```python
from build123d import *

# Parameters (mm, degrees)
BOSS_EXTRUDE1_DEPTH = 115
SKETCH2_R           = 2
CUT_EXTRUDE1_DEPTH  = 243.744721879
SKETCH3_R           = 15.5
CUT_EXTRUDE2_DEPTH  = 60


with BuildPart() as part:
    # Sketch1 → Boss-Extrude1 (new body)
    with BuildSketch(Plane.XY):
        Polygon((0, 0), (0, 40), (-5, 40), (-5, -210), (35, -210), (35, 0), align=None)
    extrude(amount=BOSS_EXTRUDE1_DEPTH)

    # Sketch2 → Cut-Extrude1 (cut, through all)
    with BuildSketch(Plane.ZY.offset(5)):
        with Locations(Location((106, 34, 0), (0, 0, 270))):
            Circle(SKETCH2_R)
        with Locations(Location((66, 34, 0), (0, 0, 270))):
            Circle(SKETCH2_R)
        with Locations((66, 6)):
            Circle(SKETCH2_R)
        with Locations((106, 6)):
            Circle(SKETCH2_R)
    extrude(amount=-CUT_EXTRUDE1_DEPTH, mode=Mode.SUBTRACT)

    # Sketch3 → Cut-Extrude2 (cut)
    with BuildSketch(Plane(origin=(0, 0, 0), x_dir=(-1, 0, 0), z_dir=(0, 0, -1))):
        with Locations((-12, 20)):
            Circle(SKETCH3_R)
    extrude(amount=-CUT_EXTRUDE2_DEPTH, mode=Mode.SUBTRACT)


solid = part.part
```
Model file for the job. Use its own axes, mm. A direction names the side the tool comes from. Give positions to 0.01 mm unless a question says otherwise; leave off trailing zeros. Write each loop counter-clockwise with the first axis right and the second up, starting at its lowest first coordinate (ties: lowest second). Pieces come first, ordered by that corner, then holes. Notation, with made-up numbers: (25.5, -2) - (53.5, -2) arc R13 cw to (53.5, 18) - close; hole circle Ø1 at (-14, 68.5). An arc over 180 degrees is marked (long way). One line per question, with ' | ' between items. Start each with the question number.
(1) Pin check, flat tips, straight feed: P1, Ø17.5, axis at x = 14, z = 43, coming from the +Y side; P2, Ø5, axis at y = 34, z = 106, coming from the +X side; P3, Ø12, axis at y = 18.5, z = 49, coming from the +X side; P4, Ø2.5, axis at y = 6, z = 66, coming from the -X side. Stop position of each tip, or through.
(2) Two-plate mould, pull along Y, no slides. Class faces 3 (the face through (-3.5, 19.9, 29.6)), 4 (the face through (-2, 40, 57)), 5 (the face through (15, -111, 0)): +Y half, -Y half, draft (parallel to the pull), parting line (faces both ways), or undercut.
(3) 3-axis set-ups, long thin cutter, end or side, ignore diameter. For faces 1 (the face through (18, 0, 57)), 2 (the face through (35, -106, 57)): which of +Z, -Z, +X, -X, +Y, -Y reach the whole face in a straight line?
(4) Slice it at A-A on z = 54.5. Write the cut outline in (x, y).
(5) Slice it at B-B on x = 24.5. Write the cut outline in (y, z), plus the area to 4 significant figures.
(6) Wall check: line 1 along Z through (x, y) = (-2.2, 34); line 2 along Y through (x, z) = (-1, 107.5); line 3 along Y through (x, z) = (5.5, 87). Give the ranges that are in metal, low to high. Write a range as from..to.
Results below:
1) P1: y = 0 | P2: x = 0 | P3: x = -1.56 | P4: through
2) face 3: undercut | face 4: +Y half | face 5: draft
3) face 1: +Z, -Z, +X, +Y | face 2: +Z, -Z, +X, +Y, -Y
4) outline: (-5, -210) - (35, -210) - (35, 0) - (0, 0) - (0, 10.19) arc R15.5 cw to (0, 29.81) - (0, 40) - (-5, 40) - close
5) outline: (-210, 0) - (0, 0) - (0, 115) - (-210, 115) - close | area: 24,150 mm^2
6) line 1: 0..64, 68..104, 108..115 | line 2: -210..4.68, 7.32..32.68, 35.32..40 | line 3: -210..0
